Read the model definition and answer for the solid it produces. Units are mm, in the model's axes. Face numbers are marked on the shaded views. A direction names the side the tool comes from. Coordinates: 2 decimals unless noted, no trailing zeros. Write each loop counter-clockwise with the first axis right and the second up, starting at its lowest first coordinate (ties: lowest second). Pieces come first, ordered by that corner, then holes. Notation, with made-up numbers: (37.5, 84) -> (50.5, 84) arc R13 ccw to (50.5, 88) -> close; hole circle Ø8 at (52.5, 16). An arc over 180 degrees is marked (long way). Use CSV: the item, a comma, the result in double quotes. Start each with the question number.
from build123d import *

# Parameters (mm, degrees)
SKETCH1_W           = 30
SKETCH1_H           = 30
BOSS_EXTRUDE1_DEPTH = 100
SKETCH2_W           = 35
SKETCH2_H           = 35
BOSS_EXTRUDE2_DEPTH = 35
SKETCH3_R           = 15
CUT_EXTRUDE1_DEPTH  = 30
SKETCH4_W           = 20
SKETCH4_H           = 20
BOSS_EXTRUDE3_DEPTH = 30


with BuildPart() as part:
    # Sketch1 → Boss-Extrude1 (new body)
    with BuildSketch(Plane(origin=(0, 0, 0), x_dir=(0, 0, -1), z_dir=(1, 0, 0))):
        Rectangle(SKETCH1_W, SKETCH1_H)
    extrude(amount=BOSS_EXTRUDE1_DEPTH)

    # Sketch2 → Boss-Extrude2 (add)
    with BuildSketch(Plane(origin=(100, 0, 0), x_dir=(0, 0, -1), z_dir=(1, 0, 0))):
        Rectangle(SKETCH2_W, SKETCH2_H)
    extrude(amount=BOSS_EXTRUDE2_DEPTH)

    # Sketch3 → Cut-Extrude1 (cut)
    with BuildSketch(Plane(origin=(135, 0, 0), x_dir=(0, 0, -1), z_dir=(1, 0, 0))):
        Circle(SKETCH3_R)
    extrude(amount=-CUT_EXTRUDE1_DEPTH, mode=Mode.SUBTRACT)

    # Sketch4 → Boss-Extrude3 (add)
    with BuildSketch(Plane(origin=(0, 17.5, 0), x_dir=(1, 0, 0), z_dir=(0, 1, 0))):
        with Locations((117.5, 0)):
            Rectangle(SKETCH4_W, SKETCH4_H)
    extrude(amount=BOSS_EXTRUDE3_DEPTH)


solid = part.part
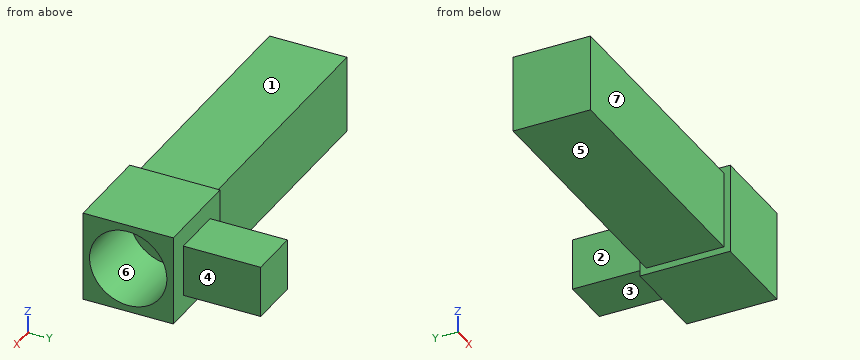
1) Which of the six approach directions +Z, -Z, +X, -X, +Y, -Y give full straight-line access (tool end or side, diameter ignored) to the marked faces 1, 2, 3 and 4?
2) Section D-D, the plane z = 5.5 is taken. Give the vertices of the cut face in (x, y), plus the area to 3 significant figures.
3) Section A-A, the plane z = 0 is taken. Give the vertices of the cut face in (x, y).
4) Find the intervals of material crossed by line 1 along Y through (x, z) = (125, 0); line 2 along Y through (x, z) = (30, -5.5), in increasing order.
5) The mould has two halves that part along Z. Classify the marked faces 5, 6 and 7: pulls with the +Z half, pulls with the -Z half, needs draft (parallel to the pull), parting line crosses it, or undercut.
6) Section B-B, the plane y = 0 is taken. Give the vertices of the cut face in (x, z).
7) Section C-C, the plane x = 88 is taken. Give the vertices of the cut face in (y, z), plus the area to 3 significant figures.
8) Each of these flat-tipped pins is pushed along its axis until it touches: pin 1 (6 mm diameter, centred on x = 59, z = 6, fed in from -Y); pin 2 (12 mm diameter, centred on y = 32, z = 1, fed in from -X); pin 3 (4 mm diameter, centred on x = 69.5, y = 15.5, fed in from -Z). Where does it stop, or does it pass through?
The answers:
1,face 1,"+Z, -X, +Y, -Y"
1,face 2,"+Z, -Z, -X, +Y"
1,face 3,"-Z, +X, -X, +Y"
1,face 4,"+Z, -Z, +X, +Y"
2,outline,"(0, -15) -> (100, -15) -> (100, -17.5) -> (135, -17.5) -> (135, -13.96) -> (105, -13.96) -> (105, 13.96) -> (135, 13.96) -> (135, 17.5) -> (127.5, 17.5) -> (127.5, 47.5) -> (107.5, 47.5) -> (107.5, 17.5) -> (100, 17.5) -> (100, 15) -> (0, 15) -> close"
2,area,"3,990 mm^2"
3,outline,"(0, -15) -> (100, -15) -> (100, -17.5) -> (135, -17.5) -> (135, -15) -> (105, -15) -> (105, 15) -> (135, 15) -> (135, 17.5) -> (127.5, 17.5) -> (127.5, 47.5) -> (107.5, 47.5) -> (107.5, 17.5) -> (100, 17.5) -> (100, 15) -> (0, 15) -> close"
4,line 1,"y = -17.5 to -15, 15 to 47.5"
4,line 2,"y = -15 to 15"
5,face 5,"pulls with the -Z half"
5,face 6,"undercut"
5,face 7,"needs draft"
6,outline,"(0, -15) -> (100, -15) -> (100, -17.5) -> (135, -17.5) -> (135, -15) -> (105, -15) -> (105, 15) -> (135, 15) -> (135, 17.5) -> (100, 17.5) -> (100, 15) -> (0, 15) -> close"
7,outline,"(-15, -15) -> (15, -15) -> (15, 15) -> (-15, 15) -> close"
7,area,"900 mm^2"
8,pin 1,"stops at y = -15"
8,pin 2,"stops at x = 107.5"
8,pin 3,"stops at z = -15"
